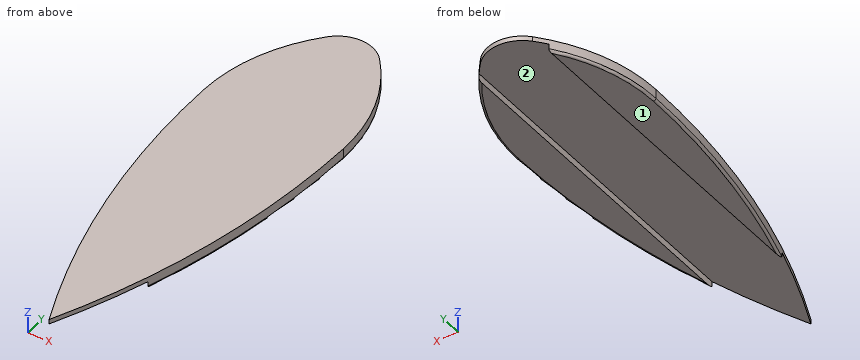
```python
from build123d import *

# Parameters (mm, degrees)
F1_DEPTH      = 25
F2_R          = 75
F3_R          = 5
F4_W          = 150
F4_H          = 30
F5_DEPTH      = 473.4323484298
F5_DEPTH_BACK = 500.0010001


with BuildPart() as f1:
    # F0 (on Top) → F1 (new body)
    with BuildSketch(Plane.XY):
        with BuildLine():
            ThreePointArc((150, 200), (110.410196625, 367.7050983125), (0, 500))
            ThreePointArc((0, 500), (-110.410196625, 367.7050983125), (-150, 200))
            ThreePointArc((-150, 200), (-112.0791240489, -157.9455265819), (0, -500))
            ThreePointArc((0, -500), (112.0791240489, -157.9455265819), (150, 200))
        make_face()
    extrude(amount=F1_DEPTH)

    # F2
    f2_edges = [f1.edges().sort_by_distance(p)[0] for p in [
        (0, 500, 12.5),
    ]]
    fillet(f2_edges, radius=F2_R)

    # F3
    f3_edges = [f1.edges().sort_by_distance(p)[0] for p in [
        (125.78038, 332.582521, 0),
        (0, 473.431348, 0),
        (112.079124, -157.945527, 0),
        (-125.78038, 332.582521, 0),
        (-112.079124, -157.945527, 0),
    ]]
    fillet(f3_edges, radius=F3_R)

    # F4 (on Front) → F5 (cut, two sides)
    with BuildSketch(Plane.XZ) as f5_sk:
        Rectangle(F4_W, F4_H)
    extrude(amount=-F5_DEPTH, mode=Mode.SUBTRACT)
    extrude(f5_sk.sketch, amount=F5_DEPTH_BACK, mode=Mode.SUBTRACT)


solid = f1.part
```
For this review, take the finished solid that the model builds, in its own axes (mm). Face numbers are marked on the shaded views. Give positions to 0.01 mm unless a question says otherwise; leave off trailing zeros. Order: outer loops, then holes, each group sorted by start corner. A loop starts at its lowest first (then second) coordinate and runs counter-clockwise, first axis right, second up.
1) The part is to be moulded in two halves that separate along X. For the marked faces 1 and 2, say which applies: released by +X, released by -X, zero draft, split by the parting line, or undercut.
2) Insertion check: pin 1 (6 mm diameter, centred on x = -75, y = 195, fed in from -Z); pin 2 (12 mm diameter, centred on y = -109.5, z = 8, fed in from +X); pin 3 (1 mm diameter, centred on x = -91.5, z = 22, fed in from +Y); pin 4 (1.5 mm diameter, centred on x = -80, z = 7.5, fed in from +Y). Each pin has a flat end and moves straight along its axis. Give the tip position at first contact, or say it passes through.
3) Take a section at A-A (x = -65.5). Give the boundary of the cut face in (y, z), then the cut area to 3 significant figures.
4) Wall thickness on line 1 (Z direction, x = 11.5, y = 196.5); line 2 (X direction, y = 337, z = 4); line 3 (X direction, y = -283, z = 3.5): over which ranges is each line inside the solid? List them lowest first.
Derived:
1. face 1: zero draft
1. face 2: undercut
2. pin 1: stops at z = 0
2. pin 2: stops at x = 122.82
2. pin 3: stops at y = 401.91
2. pin 4: stops at y = 419.22
3. outline: (-330.63, 15) - (437.14, 15) - (437.14, 25) - (-330.63, 25) - close
3. area: 7,680 mm2
4. line 1: z = 15 to 25
4. line 2: x = -123.97 to -75, 75 to 123.97
4. line 3: x = -80.06 to -75, 75 to 80.06
